Source: CAD feature listing. Evaluate the final solid. Frame: model axes, mm. A direction names the side the tool comes from. Give positions to 0.01 mm unless a question says otherwise; leave off trailing zeros. Order: outer loops, then holes, each group sorted by start corner. A loop starts at its lowest first (then second) coordinate and runs counter-clockwise, first axis right, second up. Notation, with made-up numbers: M 63,43.25 L 115,43.25 A23 ccw 115,72.25 Z; hole C 42,-9.75 d1. An arc over 180 degrees is marked long. Return JSON: item names as keys, results as strings.
from build123d import *

# Parameters (mm, degrees)
SKETCH1_W           = 14.732
SKETCH1_H           = 8.636
BOSS_EXTRUDE1_DEPTH = 1.27
SKETCH2_R           = 0.4064
BOSS_EXTRUDE2_DEPTH = 2.54
FILLET1_R           = 0.5


with BuildPart() as part:
    # Sketch1 → Boss-Extrude1 (new, symmetric)
    with BuildSketch(Plane(origin=(0, 0, 0), x_dir=(0, 0, -1), z_dir=(1, 0, 0))):
        Rectangle(SKETCH1_W, SKETCH1_H)
    extrude(amount=BOSS_EXTRUDE1_DEPTH, both=True)

    # Sketch2 → Boss-Extrude2 (add)
    with BuildSketch(Plane.XZ.offset(4.318)):
        with Locations(Location((0, 5.08, 0), (0, 0, 90))):
            Circle(SKETCH2_R)
    boss_extrude2 = extrude(amount=BOSS_EXTRUDE2_DEPTH)

    # Mirror1: Boss-Extrude2 across plane
    add(boss_extrude2.mirror(Plane.XY))

    # Fillet1
    fillet1_edges = [part.edges().sort_by_distance(p)[0] for p in [
        (1.27, 0, 7.366),
        (1.27, -4.318, 0),
        (1.27, 0, -7.366),
        (-1.27, -4.318, 0),
        (-1.27, 0, 7.366),
        (-1.27, 4.318, 0),
        (-1.27, 0, -7.366),
        (0, -4.318, -7.366),
        (0, -4.318, 7.366),
        (0, 4.318, 7.366),
        (0, 4.318, -7.366),
        (1.27, 4.318, 0),
    ]]
    fillet(fillet1_edges, radius=FILLET1_R)


solid = part.part
1. Ray query, probe 1 along Y at (x, z) = (0, 2.25); probe 2 along X at (y, z) = (4, -5); probe 3 along Z at (x, y) = (0.95, -2). Return the intervals inside material, ascending.
Evaluation:
{"probe 1": "y = -4.32 to 4.32", "probe 2": "x = -1.24 to 1.24", "probe 3": "z = -7.33 to 7.33"}
2. Draft query along Z for faces 1 (the face through (0, 0, 7.366)), 2 (the face through (-1.27, 0, 0)), 3 (the face through (0, 0, -7.366)), 4 (the face through (-0.018, -5.57, -4.674)). Return one class per face: pulls with the +Z half, pulls with the -Z half, needs draft (parallel to the pull), parting line crosses it, or undercut.
Evaluation:
{"face 1": "pulls with the +Z half", "face 2": "needs draft", "face 3": "pulls with the -Z half", "face 4": "undercut"}
3. First-contact query: pin 1 (0.8 mm diameter, centred on x = 0.5, z = 0, fed in from -Y). Flat tip, straight axial feed; report the tip coordinate or a pass-through.
Evaluation:
{"pin 1": "stops at y = -4.32"}
4. Section query A-A (z = 6.5). Return loops of the section in (x, y).
Evaluation:
{"outline": "M -1.27,-3.82 A0.5 ccw -0.77,-4.32 L 0.77,-4.32 A0.5 ccw 1.27,-3.82 L 1.27,3.82 A0.5 ccw 0.77,4.32 L -0.77,4.32 A0.5 ccw -1.27,3.82 Z"}
5. Set-up query: faces 5 (the face through (0, -6.858, -5)), 6 (the face through (-0.018, -5.57, 4.674)). Return all of +Z, -Z, +X, -X, +Y, -Y with unobstructed straight access to the full face (end or side cutting, diameter ignored); none if empty.
Evaluation:
{"face 5": "+Z, -Z, +X, -X, -Y", "face 6": "-Y"}
6. Section query B-B (x = 0). Return loops of the section in (y, z).
Evaluation:
{"outline": "M -6.86,-5.49 L -4.32,-5.49 L -4.32,-6.87 A0.5 ccw -3.82,-7.37 L 3.82,-7.37 A0.5 ccw 4.32,-6.87 L 4.32,6.87 A0.5 ccw 3.82,7.37 L -3.82,7.37 A0.5 ccw -4.32,6.87 L -4.32,5.49 L -6.86,5.49 L -6.86,4.67 L -4.32,4.67 L -4.32,-4.67 L -6.86,-4.67 Z"}
